Autodesk Inventor part; units mm, degrees
ref_plane "YZ Plane" through (0, 0, 0) normal (1, 0, 0) x (0, 1, 0)
ref_plane "XZ Plane" through (0, 0, 0) normal (0, 1, 0) x (-1, 0, 0)
ref_plane "XY Plane" through (0, 0, 0) normal (0, 0, 1) x (1, 0, 0)
sketch "Sketch1" plane through (0, 0, 0) normal (0, 0, 1) x (1, 0, 0)
  line L0 (-6.4008, -4.6609) -> (6.4008, -4.6609)
  line L1 (6.4008, -4.6609) -> (6.4008, 4.6609)
  line L2 (6.4008, 4.6609) -> (-6.4008, 4.6609)
  line L3 (-6.4008, 4.6609) -> (-6.4008, -4.6609)
  line L4 (-6.4008, -4.6609) -> (6.4008, 4.6609) construction
  line L5 (6.4008, -4.6609) -> (-6.4008, 4.6609) construction
  point P0 (0, 0)
  dimension "d0" = 12.8016
  dimension "d1" = 9.3218
extrude "Extrusion1" add sketch "Sketch1" along normal blind 6.35
sketch "Sketch2" plane through (-6.4008, 4.6609, 0) normal (0, 1, 0) x (1, 0, 0)
  line L0 (0, 0) -> (0, -6.35)
  line L1 (12.8016, 0) -> (12.8016, -6.35)
  line L2 (0, -6.35) -> (12.8016, -6.35)
  circle A0 centre (6.4008, -3.175) radius 2.8575
  point P0 (6.4008, 0)
  dimension "d4" = 5.715
extrude "Extrusion2" add sketch "Sketch2" along normal blind 5.08
sketch "Sketch3" plane through (0, 9.7409, 3.175) normal (0, 1, 0) x (1, 0, 0)
  circle A0 centre (0, 0) radius 1.397
  point P0 (0, 3.175)
  dimension "d7" = 2.794
extrude "Extrusion3" add sketch "Sketch3" along normal blind 5.08
properties part number "switch jp"
Build history of the part. All positions in model axes, mm. A direction names the side the tool comes from. Give positions to 0.01 mm unless a question says otherwise; leave off trailing zeros. Loops run counter-clockwise (first coordinate to the right, second up) from the corner with the lowest first, then second, coordinate; pieces in that order, holes last.
1) Band-saw the part on B-B on z = 1. List the corners of the cut face in (x, y).
Values follow:
outline: (-6.4, -4.66) - (6.4, -4.66) - (6.4, 4.66) - (1.85, 4.66) - (1.85, 9.74) - (-1.85, 9.74) - (-1.85, 4.66) - (-6.4, 4.66) - close
2) Probe line 1 along Y through (x, z) = (5, 0.5); line 2 along Y through (x, z) = (0.75, 4.75); line 3 along Z through (x, y) = (1.5, 5.75). List the from-to ranges inside material, lowest first.
Values follow:
line 1: y = -4.66 to 4.66
line 2: y = -4.66 to 9.74
line 3: z = 0.74 to 5.61
3) Band-saw the part on C-C on z = 3.5. List the corners of the cut face in (x, y), then the cut area to 3 significant figures.
Values follow:
outline: (-6.4, -4.66) - (6.4, -4.66) - (6.4, 4.66) - (2.84, 4.66) - (2.84, 9.74) - (1.36, 9.74) - (1.36, 14.82) - (-1.36, 14.82) - (-1.36, 9.74) - (-2.84, 9.74) - (-2.84, 4.66) - (-6.4, 4.66) - close
area: 162 mm2
4) Two-plate mould, pull along Z, no slides. Class faces 1 (the face through (3, 4.661, 2)), 2 (the face through (-0.18, 12.25, 4.56)), 3 (the face through (0, 0, 6.35)): released by +Z, released by -Z, zero draft, split by the parting line, or undercut.
Values follow:
face 1: zero draft
face 2: split by the parting line
face 3: released by +Z
5) Band-saw the part on A-A on x = 0. List the corners of the cut face in (y, z), then the cut area to 3 significant figures.
Values follow:
outline: (-4.66, 0) - (4.66, 0) - (4.66, 0.32) - (9.74, 0.32) - (9.74, 1.78) - (14.82, 1.78) - (14.82, 4.57) - (9.74, 4.57) - (9.74, 6.03) - (4.66, 6.03) - (4.66, 6.35) - (-4.66, 6.35) - close
area: 102 mm2
6) Band-saw the part on D-D on x = 4. List the corners of the cut face in (y, z).
Values follow:
outline: (-4.66, 0) - (4.66, 0) - (4.66, 6.35) - (-4.66, 6.35) - close
7) 3-axis set-ups, long thin cutter, end or side, ignore diameter. For faces 4 (the face through (0, 14.821, 3)), 5 (the face through (-2.27, 7.17, 1.44)): which of +Z, -Z, +X, -X, +Y, -Y reach the whole face in a straight line?
Values follow:
face 4: +Z, -Z, +X, -X, +Y
face 5: +Y
8) Drop a flat-ended pin along its axis: P1, Ø2, axis at x = 5, z = 1.5, coming from the +Y side. Give the stop position or say it passes through.
Values follow:
P1: stops at y = 4.66
